from build123d import *

# Parameters (mm, degrees)
SKETCH1_R           = 7.5
BOSS_EXTRUDE1_DEPTH = 29.788449
SKETCH2_R           = 3.684354477
CUT_EXTRUDE1_DEPTH  = 32.620431588
CHAMFER1_SIZE       = 0.93743


with BuildPart() as part:
    # Sketch1 → Boss-Extrude1 (new body)
    with BuildSketch(Plane(origin=(0, 0, 0), x_dir=(1, 0, 0), z_dir=(0, 1, 0))):
        with Locations(Location((0, 0, 0), (0, 0, 270))):
            Circle(SKETCH1_R)
    extrude(amount=BOSS_EXTRUDE1_DEPTH)

    # Sketch2 → Cut-Extrude1 (cut, through all)
    with BuildSketch(Plane(origin=(0, 0, 0), x_dir=(1, 0, 0), z_dir=(0, 1, 0))):
        with Locations(Location((0, 0, 0), (0, 0, 270))):
            Circle(SKETCH2_R)
    extrude(amount=CUT_EXTRUDE1_DEPTH, mode=Mode.SUBTRACT)

    # Chamfer1
    chamfer1_edges = [part.edges().sort_by_distance(p)[0] for p in [
        (0, 0, -7.5),
        (0, 29.788449, -7.5),
        (0, 0, -3.684354477),
        (0, 29.788449, -3.684354477),
    ]]
    chamfer(chamfer1_edges, length=CHAMFER1_SIZE)


solid = part.part
Could you check a few things on this model? Use its own coordinates, in mm. Coordinates: 2 decimals unless noted, no trailing zeros. Order: outer loops, then holes, each group sorted by start corner. A loop starts at its lowest first (then second) coordinate and runs counter-clockwise, first axis right, second up. Notation, with made-up numbers: (-31, -5.5) -> (28, -5.5) arc R21 cw to (28, 21.5) -> close; hole circle Ø2 at (85, 62). An arc over 180 degrees is marked (long way). One line per item, written item: value. Start each with the question number.
1) Imagine slicing it at A-A on z = 0. List the corners of the cut face in (x, y) for me.
2) Imagine slicing it at C-C on y = 11.5. List the corners of the cut face in (x, z) for me.
3) We'd pull the mould along Z, two halves only. Please class faces 1 (the cylindrical face through (3.653, 14.699, -0.48)), 2 (the flat face through (4.5, 0, -1.6)), 3 (the cylindrical face through (0.33, 14.699, -7.493)): +Z half, -Z half, draft (parallel to the pull), parting line (faces both ways), or undercut.
4) Imagine slicing it at B-B on x = 0. List the corners of the cut face in (y, z) for me.
5) If I drill on L1, parallel to X at y = 12, z = 0; L2, parallel to Z at x = 1.25, y = 4; L3, parallel to Z at x = -2.5, y = 17, over which ranges is the centre line in solid material (lowest first)? Write a range as [from, to].
6) I'm going to push flat-ended pins straight in: pin 1 (4 mm diameter, centred on y = 22.5, z = 2.5, fed in from -X); pin 2 (3 mm diameter, centred on y = 18, z = -6, fed in from +X); pin 3 (1.5 mm diameter, centred on x = 6, y = 19.5, fed in from +Z). Where does each tip first touch, or does it pass through?
Answer list:
1. outline: (-7.5, 0.94) -> (-6.56, 0) -> (-4.62, 0) -> (-3.68, 0.94) -> (-3.68, 28.85) -> (-4.62, 29.79) -> (-6.56, 29.79) -> (-7.5, 28.85) -> close; (3.68, 0.94) -> (4.62, 0) -> (6.56, 0) -> (7.5, 0.94) -> (7.5, 28.85) -> (6.56, 29.79) -> (4.62, 29.79) -> (3.68, 28.85) -> close
2. outline: circle Ø15 at (0, 0); hole circle Ø7.37 at (0, 0)
3. face 1: undercut
3. face 2: draft
3. face 3: parting line
4. outline: (0, -6.56) -> (0.94, -7.5) -> (28.85, -7.5) -> (29.79, -6.56) -> (29.79, -4.62) -> (28.85, -3.68) -> (0.94, -3.68) -> (0, -4.62) -> close; (0, 4.62) -> (0.94, 3.68) -> (28.85, 3.68) -> (29.79, 4.62) -> (29.79, 6.56) -> (28.85, 7.5) -> (0.94, 7.5) -> (0, 6.56) -> close
5. L1: x = [-7.5, -3.68], [3.68, 7.5]
5. L2: z = [-7.4, -3.47], [3.47, 7.4]
5. L3: z = [-7.07, -2.71], [2.71, 7.07]
6. pin 1: stops at x = -7.48
6. pin 2: stops at x = 6
6. pin 3: stops at z = 5.36
